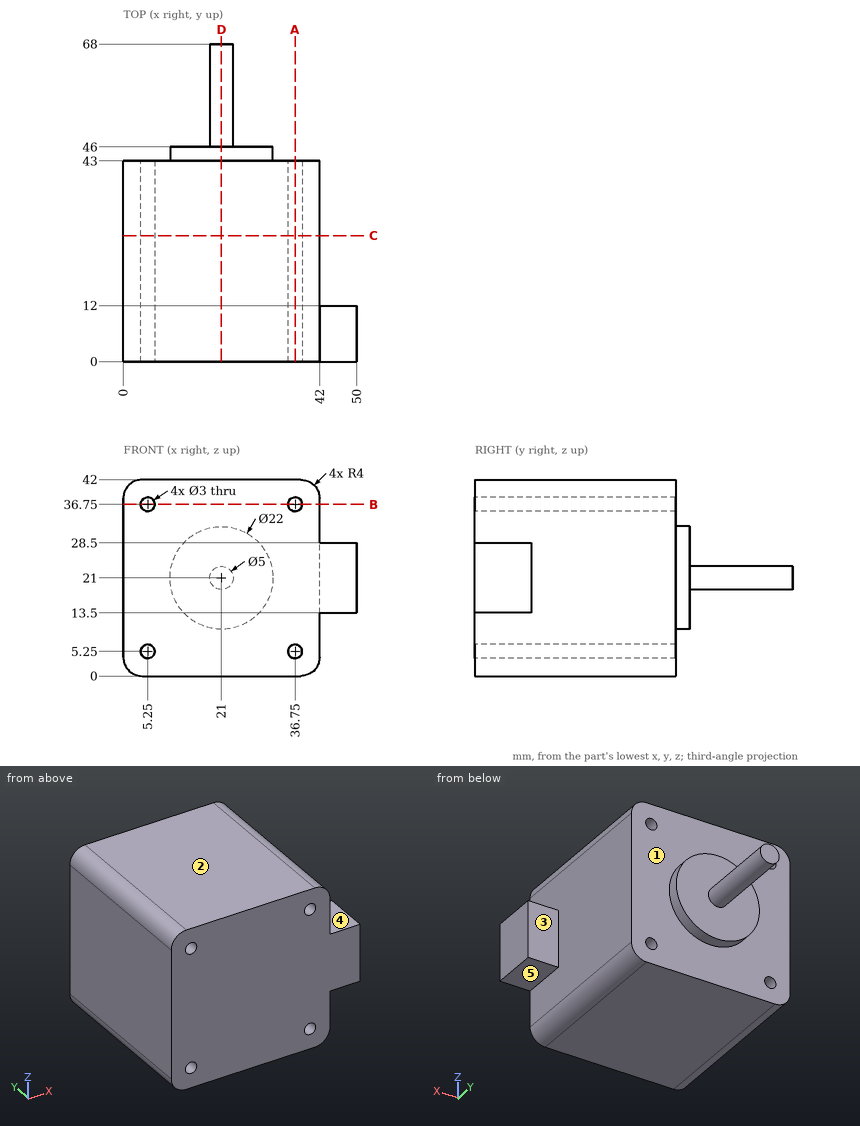
Print and shaded views of the part. All mm, measured from the part's lowest x, y and z. A direction names the side the tool comes from. Coordinates: 2 decimals unless noted, no trailing zeros. Order: outer loops, then holes, each group sorted by start corner. A loop starts at its lowest first (then second) coordinate and runs counter-clockwise, first axis right, second up. Notation, with made-up numbers: (62, 8.5) - (68, 8.5) arc R29 ccw to (68, 41.5) - close; hole circle Ø2 at (12, -31.75). An arc over 180 degrees is marked (long way). Return JSON: item names as keys, results as strings. Group by question number.
Item 1: Drill centre lines: probe 1 along X at (y, z) = (28.5, 36.75); probe 2 along X at (y, z) = (16, 36). Where is each one in solid material? Low to high. Write a range as from..to.
Item 2: Which spindle directions (+Z, -Z, +X, -X, +Y, -Y) get a long thin tool onto all of the face, cutting with end or side? Do the marked faces 1, 2, 3, 4 and 5. Say none if no direction does.
Item 3: Cut at C-C (y = 27). List the corners of the cut face in (x, z), plus the area to 3 significant figures.
Item 4: Cut at D-D (x = 21). List the corners of the cut face in (y, z).
Item 5: Cut at B-B (z = 36.75). List the corners of the cut face in (x, y), plus the area to 3 significant figures.
Item 6: Cut at A-A (x = 36.75). List the corners of the cut face in (y, z), plus the area to 3 significant figures.
Item 7: Pin check, flat tips, straight feed: pin 1 (3 mm diameter, centred on x = 19, z = 35.5, fed in from +Y); pin 2 (10 mm diameter, centred on y = 58, z = 16, fed in from -X); pin 3 (2.5 mm diameter, centred on x = 46, y = 6.5, fed in from -Z); pin 4 (3 mm diameter, centred on x = 25, y = 13, fed in from -Z). Stop position of each tip, or through.
Check values:
{
 "1": {"probe 1": "x = 0..3.75, 6.75..35.25, 38.25..42", "probe 2": "x = 0..3.95, 6.55..35.45, 38.05..42"},
 "2": {"face 1": "+Y", "face 2": "+Z, +X, -X, +Y, -Y", "face 3": "+Z, -Z, +X, +Y", "face 4": "+Z, +X, +Y, -Y", "face 5": "-Z, +X, +Y, -Y"},
 "3": {"outline": "(0, 4) arc R4 ccw to (4, 0) - (38, 0) arc R4 ccw to (42, 4) - (42, 38) arc R4 ccw to (38, 42) - (4, 42) arc R4 ccw to (0, 38) - close; hole circle Ø3 at (5.25, 5.25); hole circle Ø3 at (5.25, 36.75); hole circle Ø3 at (36.75, 5.25); hole circle Ø3 at (36.75, 36.75)", "area": "1,720 mm2"},
 "4": {"outline": "(0, 0) - (43, 0) - (43, 10) - (46, 10) - (46, 18.5) - (68, 18.5) - (68, 23.5) - (46, 23.5) - (46, 32) - (43, 32) - (43, 42) - (0, 42) - close"},
 "5": {"outline": "(0, 0) - (3.75, 0) - (3.75, 43) - (0, 43) - close; (6.75, 0) - (35.25, 0) - (35.25, 43) - (6.75, 43) - close; (38.25, 0) - (42, 0) - (42, 43) - (38.25, 43) - close", "area": "1,550 mm2"},
 "6": {"outline": "(0, 0) - (43, 0) - (43, 3.75) - (0, 3.75) - close; (0, 6.75) - (43, 6.75) - (43, 35.25) - (0, 35.25) - close; (0, 38.25) - (43, 38.25) - (43, 42) - (0, 42) - close", "area": "1,550 mm2"},
 "7": {"pin 1": "stops at y = 43", "pin 2": "stops at x = 18.5", "pin 3": "stops at z = 13.5", "pin 4": "stops at z = 0"}
}
